Autodesk Inventor part; units mm, degrees
sketch "Boceto1" plane through (0, 0, 0) normal (0, 0, 1) x (1, 0, 0)
  line L0 (0, 0) -> (107, 0)
  line L1 (107, 0) -> (107, -5.5)
  line L2 (107, -5.5) -> (82, -30.4995)
  line L3 (82, -30.4995) -> (12, -30.4995)
  line L4 (12, -30.4995) -> (-13, -5.5)
  line L5 (-13, -5.5) -> (-13, 27)
  line L6 (-13, 27) -> (0, 27)
  line L7 (0, 27) -> (0, 0)
  dimension "d0" = 107
  dimension "d1" = 5.5
  dimension "d2" = 35.355
  dimension "d3" = 70
  dimension "d4" = 35.355
  dimension "d5" = 32.5
  dimension "d6" = 13
  dimension "d7" = 27
extrude "Extrusión1" add sketch "Boceto1" along normal blind 10
sketch "Boceto2" plane through (0, 0, 10) normal (0, 0, 1) x (1, 0, 0)
  circle A0 centre (22, -5.4995) radius 1.89
  circle A1 centre (47, -5.4995) radius 1.89
  circle A2 centre (72, -5.4995) radius 1.89
  circle A3 centre (-5.5, 12) radius 1.89
  circle A4 centre (22, -22.7495) radius 1.89
  circle A5 centre (72, -22.7495) radius 1.89
  line L0 (12, -30.4995) -> (82, -30.4995)
  line L1 (-13, 27) -> (-13, -5.5)
  line L2 (0, 27) -> (-13, 27)
  line L3 (0, 27) -> (0, 0)
  dimension "d10" = 3.78
  dimension "d11" = 3.78
  dimension "d12" = 3.78
  dimension "d13" = 3.78
  dimension "d14" = 3.78
  dimension "d15" = 3.78
  dimension "d16" = 25
  dimension "d17" = 25
  dimension "d18" = 17.25
  dimension "d19" = 7.75
  dimension "d20" = 35
  dimension "d21" = 15
  dimension "d22" = 5.5
extrude "Extrusión2" cut sketch "Boceto2" against normal through all
sketch "Boceto3" plane through (0, 0, 0) normal (0, 0, -1) x (-1, 0, 0)
  circle A0 centre (-72, -22.7495) radius 1.89
  circle A1 centre (-22, -22.7495) radius 1.89
  circle A2 centre (-72, -22.7495) radius 3.6
  circle A3 centre (-22, -22.7495) radius 3.6
  point P0 (0, 0)
  dimension "d25" = 7.2
  dimension "d26" = 7.2
extrude "Extrusión3" cut sketch "Boceto3" against normal blind 2.79
ref_plane "Plano de trabajo1" through (0, 0, 5.61) normal (0, 0, 1) x (1, 0, 0)
sketch "Boceto4" plane through (0, 0, 5.61) normal (0, 0, 1) x (1, 0, 0)
  circle A0 centre (-5.5, 12) radius 1.89
  circle A1 centre (22, -5.4995) radius 1.89
  circle A2 centre (47, -5.4995) radius 1.89
  circle A3 centre (72, -5.4995) radius 1.89
  line L0 (0, 27) -> (0, 0)
  line L1 (0, 15.1175) -> (-7.3, 15.1175)
  line L2 (-7.3, 15.1175) -> (-9.1003, 12)
  line L3 (-9.1003, 12) -> (-7.3, 8.8825)
  line L4 (-7.3, 8.8825) -> (0, 8.8825)
  line L5 (0, 15.1175) -> (0, 8.8825)
  line L6 (22, -9.1003) -> (18.8825, -7.3)
  line L7 (18.8825, -7.3) -> (18.8825, 0)
  line L8 (0, 0) -> (107, 0)
  line L9 (22, -9.1003) -> (25.1175, -7.3)
  line L10 (25.1175, -7.3) -> (25.1175, 0)
  line L11 (25.1175, 0) -> (18.8825, 0)
  point P0 (0, 12)
  point P1 (22, 0)
  dimension "d30" = 7.3
  dimension "d31" = 6.235
  dimension "d32" = 3.6
  dimension "d33" = 6.235
  dimension "d34" = 3.6
  dimension "d35" = 7.3
extrude "Extrusión4" cut sketch "Boceto4" against normal blind 3 contours L8 L10 L9 L6 L7 | L0 L4 L3 L2 L1
pattern_linear "Patrón rectangular1" count 3 spacing -25 along (-1, 0, 0) of "Extrusión4"
sketch "Boceto5" plane through (0, 0, 0) normal (0, 0, -1) x (-1, 0, 0)
  line L0 (-98, 0) -> (-98, -4)
  line L1 (-98, -4) -> (4, -4)
  line L2 (4, -4) -> (4, 27)
  line L3 (13, 27) -> (0, 27)
  line L4 (0, 27) -> (4, 27)
  line L5 (0, 27) -> (0, 0)
  line L6 (0, 0) -> (0, 27)
  line L7 (0, 0) -> (-98, 0)
  line L8 (-107, 0) -> (-107, -5.5)
  line L9 (13, -5.5) -> (13, 27)
  dimension "d41" = 4
  dimension "d42" = 9
  dimension "d43" = 9
extrude "Extrusión5" cut sketch "Boceto5" against normal blind 0.8
Geometry check sheet. Reference: the model listing, model coordinates, mm. A direction names the side the tool comes from. Round coordinates to 2 decimals unless told otherwise and drop trailing zeros. Loops run counter-clockwise (first coordinate to the right, second up) from the corner with the lowest first, then second, coordinate; pieces in that order, holes last. Notation, with made-up numbers: (-15, 11.5) -> (24, 11.5) arc R30 cw to (24, 49.5) -> close; hole circle Ø4 at (5.5, 55). An arc over 180 degrees is marked (long way). Answer as a JSON object with one key per item and string values. Group by question number.
Item 1: Release check for a two-part mould opening along Y. For faces 1 (the face through (70, -24, 2.79)), 2 (the face through (36, -1, 0.8)), 3 (the face through (53, 0, 5)), 4 (the face through (45.61, -4.22, 7.84)) record: pulls with the +Y half, pulls with the -Y half, needs draft (parallel to the pull), parting line crosses it, or undercut.
Item 2: Set-up check for faces 5 (the face through (23.54, -8.21, 4.13)), 6 (the face through (-3, 12, 5.61)), 7 (the face through (20, -24, 2.79)): record each of +Z, -Z, +X, -X, +Y, -Y from which the full face is reachable in a straight line by a thin tool's end or side.
Item 3: Thickness scan on line 1 along Y through (x, z) = (72, 7.55); line 2 along Y through (x, z) = (51.5, 6.5); line 3 along X through (y, z) = (-22.5, 6.25). Record the ranges inside material, lowest first.
Item 4: Cross-section at C-C, the plane x = 62. Record the cut outline in (y, z), plus the area to 3 significant figures.
Item 5: Cross-section at B-B, the plane y = 5. Record the cut outline in (x, z), plus the area to 3 significant figures.
Item 6: Depth check by flat-ended pin: pin 1 Ø6 at (x, z) = (18.5, 5) entering from +Y; pin 2 Ø6.5 at (x, y) = (22, -22.75) entering from -Z; pin 3 Ø3 at (y, z) = (12.5, 6.5) entering from +X. Enter the tip coordinate at first touch or a pass-through.
Item 7: Cross-section at A-A, the plane x = -6. Record the cut outline in (y, z), plus the area to 3 significant figures.
Determined:
{
 "1": {"face 1": "undercut", "face 2": "needs draft", "face 3": "pulls with the +Y half", "face 4": "undercut"},
 "2": {"face 5": "+Y", "face 6": "+X", "face 7": "-Z"},
 "3": {"line 1": "y = -30.5 to -24.64, -20.86 to -7.39, -3.61 to 0", "line 2": "y = -30.5 to 0", "line 3": "x = 4 to 20.13, 23.87 to 70.13, 73.87 to 90"},
 "4": {"outline": "(-30.5, 0) -> (-4, 0) -> (-4, 0.8) -> (0, 0.8) -> (0, 10) -> (-30.5, 10) -> close", "area": "302 mm²"},
 "5": {"outline": "(-13, 0) -> (-4, 0) -> (-4, 0.8) -> (0, 0.8) -> (0, 10) -> (-13, 10) -> close", "area": "127 mm²"},
 "6": {"pin 1": "stops at y = 0", "pin 2": "stops at z = 2.79", "pin 3": "stops at x = 0"},
 "7": {"outline": "(-12.5, 0) -> (10.18, 0) -> (10.18, 2.61) -> (8.88, 2.61) -> (8.88, 5.61) -> (10.18, 5.61) -> (10.18, 10) -> (-12.5, 10) -> close; (13.82, 0) -> (27, 0) -> (27, 10) -> (13.82, 10) -> (13.82, 5.61) -> (15.12, 5.61) -> (15.12, 2.61) -> (13.82, 2.61) -> close", "area": "351 mm²"}
}
